Check sheet for the modelled part. Datum: model origin and axes. Units: mm. A direction names the side the tool comes from. Round coordinates to 2 decimals unless told otherwise and drop trailing zeros. Loops run counter-clockwise (first coordinate to the right, second up) from the corner with the lowest first, then second, coordinate; pieces in that order, holes last. Notation, with made-up numbers: (6, -3) -> (34, -3) arc R24 ccw to (34, 8) -> close; hole circle Ø8 at (17.25, 59). An arc over 180 degrees is marked (long way). One line per item, written item: value. Start each with the question number.
1. Cross-section at B-B on y = -490.5. Record the cut outline in (x, z).
2. Release check for a two-part mould opening along Y. For faces 1 (the face through (355, 0, 197)), 2 (the face through (345, -795, 205)), 3 (the face through (0, -406, 197)), 4 (the face through (5, -406, 205)) record: +Y half, -Y half, draft (parallel to the pull), parting line (faces both ways), or undercut.
3. Material ranges on L1, parallel to X at y = -247, z = 249; L2, parallel to Y at x = 202, z = 86; L3, parallel to Z at x = 106, y = -645.5, recorded low to high.
4. Go/stop test with flat-tipped pins: pin 1 (1.5 mm diameter, centred on y = -461, z = 227, fed in from +X); pin 2 (4 mm diameter, centred on x = 710, z = 407.5, fed in from +Y); pin 3 (15.5 mm diameter, centred on x = 708.5, z = 406.5, fed in from -Y). Record where each tip stops, or that it passes through.
5. Cross-section at A-A on z = 196.5. Record the cut outline in (x, y), then the cut area to 3 significant figures.
6. Set-up check for faces 5 (the face through (345, -5, 205)), 6 (the face through (355, -800, 197)): record each of +Z, -Z, +X, -X, +Y, -Y from which the full face is reachable in a straight line by a thin tool's end or side.
7. Cross-section at C-C on x = 65. Record the cut outline in (y, z).
8. Cross-section at D-D on y = -145.5. Record the cut outline in (x, z), then the cut area to 3 significant figures.
from build123d import *

# Parameters (mm, degrees)
CROQUIS1_W              = 700
CROQUIS1_H              = 800
SALIENTE_EXTRUIR1_DEPTH = 400
CROQUIS2_W              = 690
CROQUIS2_H              = 790
CORTAR_EXTRUIR1_DEPTH   = 395
SALIENTE_EXTRUIR2_DEPTH = 800
CROQUIS4_W              = 56.686989083
CROQUIS4_H              = 120
CROQUIS4_H_2            = 440
CORTAR_EXTRUIR2_DEPTH   = 450


with BuildPart() as part:
    # Croquis1 → Saliente-Extruir1 (new body)
    with BuildSketch(Plane.XY):
        with Locations((350, -400)):
            Rectangle(CROQUIS1_W, CROQUIS1_H)
    extrude(amount=SALIENTE_EXTRUIR1_DEPTH)

    # Croquis2 → Cortar-Extruir1 (cut)
    with BuildSketch(Plane.XY.offset(400)):
        with Locations((350, -400)):
            Rectangle(CROQUIS2_W, CROQUIS2_H)
    extrude(amount=-CORTAR_EXTRUIR1_DEPTH, mode=Mode.SUBTRACT)

    # Croquis3 → Saliente-Extruir2 (add)
    with BuildSketch(Plane(origin=(0, 0, 0), x_dir=(1, 0, 0), z_dir=(0, 1, 0))):
        with BuildLine():
            Line((700, -396.545914708), (706, -396.545914708))
            Line((706, -396.545914708), (710.25902772, -400.804942428))
            ThreePointArc((710.25902772, -400.804942428), (708.049920297, -413.920814068), (702.050252532, -402.050252532))
            Line((702.050252532, -402.050252532), (700, -400))
            Line((700, -400), (700, -396.545914708))
        make_face()
    extrude(amount=-SALIENTE_EXTRUIR2_DEPTH)

    # Croquis4 → Cortar-Extruir2 (cut)
    with BuildSketch(Plane(origin=(0, 0, 0), x_dir=(-1, 0, 0), z_dir=(0, 0, -1))):
        with Locations((-728.343494542, -60)):
            Rectangle(CROQUIS4_W, CROQUIS4_H)
        with Locations((-728.343494542, -740)):
            Rectangle(CROQUIS4_W, CROQUIS4_H)
        with Locations((-728.343494542, -400)):
            Rectangle(CROQUIS4_W, CROQUIS4_H_2)
    extrude(amount=-CORTAR_EXTRUIR2_DEPTH, mode=Mode.SUBTRACT)


solid = part.part
Taken from the geometry:
1. outline: (0, 0) -> (700, 0) -> (700, 400) -> (695, 400) -> (695, 5) -> (5, 5) -> (5, 400) -> (0, 400) -> close
2. face 1: +Y half
2. face 2: undercut
2. face 3: draft
2. face 4: undercut
3. L1: x = 0 to 5, 695 to 700
3. L2: y = -800 to -795, -5 to 0
3. L3: z = 0 to 5
4. pin 1: stops at x = 700
4. pin 2: stops at y = -120
4. pin 3: stops at y = -680
5. outline: (0, -800) -> (700, -800) -> (700, 0) -> (0, 0) -> close; hole (5, -795) -> (695, -795) -> (695, -5) -> (5, -5) -> close
5. area: 14,900 mm2
6. face 5: +Z
6. face 6: +Z, -Z, +X, -X, -Y
7. outline: (-800, 0) -> (0, 0) -> (0, 400) -> (-5, 400) -> (-5, 5) -> (-795, 5) -> (-795, 400) -> (-800, 400) -> close
8. outline: (0, 0) -> (700, 0) -> (700, 396.55) -> (706, 396.55) -> (710.26, 400.8) arc R7 ccw (long way) to (702.05, 402.05) -> (700, 400) -> (695, 400) -> (695, 5) -> (5, 5) -> (5, 400) -> (0, 400) -> close
8. area: 7,640 mm2
